from build123d import *

# Parameters (mm, degrees)
F2_R     = 1
F3_DEPTH = 10
F4_W     = 0.5
F4_H     = 4
F5_DEPTH = 30.001


with BuildPart() as f1:
    # F0 (on Right) → F1 (revolve)
    with BuildSketch(Plane.YZ):
        Polygon((5.690518, 7.5), (-0.309482, 7.5), (-0.309482, 5), (-10.309482, 5), (-10.309482, 0), (19.690518, 0), (19.690518, 7.5), (9.690518, 7.5), (9.690518, 4.5), (8.190518, 4.5), (8.190518, 7.5), (7.190518, 7.5), (7.190518, 4.5), (5.690518, 4.5), align=None)
    revolve(axis=Axis((0, 12.775562, 0), (0, 1, 0)))

    # F2 (on face) → F3 (cut)
    with BuildSketch(Plane.XZ.offset(10.309482)):
        with Locations((-2.5, 2)):
            Circle(F2_R)
        with Locations((2.5, 2)):
            Circle(F2_R)
        with Locations((-2.5, -2)):
            Circle(F2_R)
        with Locations((2.5, -2)):
            Circle(F2_R)
    extrude(amount=-F3_DEPTH, mode=Mode.SUBTRACT)

    # F4 (on face) → F5 (cut, through all)
    with BuildSketch(Plane.XZ.offset(10.309482)):
        with Locations((-0.25, 5.5)):
            Rectangle(F4_W, F4_H)
        with Locations((0.25, 5.5)):
            Rectangle(F4_W, F4_H)
    extrude(amount=-F5_DEPTH, mode=Mode.SUBTRACT)


solid = f1.part
Check sheet for the modelled part. Datum: model origin and axes. Units: mm. A direction names the side the tool comes from. Coordinates: 2 decimals unless noted, no trailing zeros. Write each loop counter-clockwise with the first axis right and the second up, starting at its lowest first coordinate (ties: lowest second). Pieces come first, ordered by that corner, then holes. Notation, with made-up numbers: M -21,-4.75 L 7,-4.75 A23 cw 7,11.25 Z; hole C 58.25,-39.75 d6. An arc over 180 degrees is marked long. Answer as CSV lines item,"result".
Q1. Cross-section at A-A (x = 0). Record the boundary of the cut face in (y, z), then the cut area to 3 significant figures.
Check result:
outline,"M -10.31,-5 L -0.31,-5 L -0.31,-7.5 L 5.69,-7.5 L 5.69,-4.5 L 7.19,-4.5 L 7.19,-7.5 L 8.19,-7.5 L 8.19,-4.5 L 9.69,-4.5 L 9.69,-7.5 L 19.69,-7.5 L 19.69,3.5 L -10.31,3.5 Z"
area,"296 mm^2"
Q2. Go/stop test with flat-tipped pins: pin 1 (3 mm diameter, centred on y = 9, z = 5.5, fed in from -X); pin 2 (1.6 mm diameter, centred on x = -2.5, z = -2, fed in from -Y); pin 3 (1.5 mm diameter, centred on x = 6, y = 4, fed in from +Z). Record where each tip stops, or that it passes through.
Check result:
pin 1,"x = -6.23"
pin 2,"y = -0.31"
pin 3,"z = 5.36"
Q3. Cross-section at B-B (y = -4). Record the boundary of the cut face in (x, z).
Check result:
outline,"M -0.5,3.5 L -0.5,4.97 A5 ccw long 0.5,4.97 L 0.5,3.5 Z; hole C -2.5,-2 d2; hole C -2.5,2 d2; hole C 2.5,-2 d2; hole C 2.5,2 d2"
Q4. Mould release check, pull along Y, two halves, no side actions. Record for faces 1 (the face through (-2, -0.309, 5)), 2 (the face through (-3.2, 7.191, -3.4)), 3 (the face through (-3.3, -5.4, -2.6)): released by +Y, released by -Y, zero draft, split by the parting line, or undercut.
Check result:
face 1,"released by -Y"
face 2,"undercut"
face 3,"zero draft"
Q5. Material ranges on probe 1 along Y at (x, z) = (-2.5, 4.5); probe 2 along Y at (x, z) = (1, -4.5); probe 3 along Z at (x, y) = (-2.5, -4.5), recorded low to high. Write a range as from..to.
Check result:
probe 1,"-0.31..5.69, 7.19..8.19, 9.69..19.69"
probe 2,"-10.31..5.69, 7.19..8.19, 9.69..19.69"
probe 3,"-4.33..-3, -1..1, 3..4.33"
Q6. Cross-section at D-D (z = 0). Record the boundary of the cut face in (x, y), then the cut area to 3 significant figures.
Check result:
outline,"M -7.5,-0.31 L -5,-0.31 L -5,-10.31 L 5,-10.31 L 5,-0.31 L 7.5,-0.31 L 7.5,5.69 L 4.5,5.69 L 4.5,7.19 L 7.5,7.19 L 7.5,8.19 L 4.5,8.19 L 4.5,9.69 L 7.5,9.69 L 7.5,19.69 L -7.5,19.69 L -7.5,9.69 L -4.5,9.69 L -4.5,8.19 L -7.5,8.19 L -7.5,7.19 L -4.5,7.19 L -4.5,5.69 L -7.5,5.69 Z"
area,"382 mm^2"
Q7. Set-up check for faces 4 (the face through (0.323, 2.649, -7.493)), 5 (the face through (0, 4, 3.5)), 6 (the face through (2, -0.309, -2)), 7 (the face through (-3.2, 9.691, -3.4)): record each of +Z, -Z, +X, -X, +Y, -Y from which the full face is reachable in a straight line by a thin tool's end or side.
Check result:
face 4,"+Y, -Y"
face 5,"+Z, +Y, -Y"
face 6,"-Y"
face 7,"none"
Q8. Cross-section at C-C (z = -6.5). Record the boundary of the cut face in (x, y), then the cut area to 3 significant figures.
Check result:
outline,"M -3.74,-0.31 L 3.74,-0.31 L 3.74,5.69 L -3.74,5.69 Z; M -3.74,7.19 L 3.74,7.19 L 3.74,8.19 L -3.74,8.19 Z; M -3.74,9.69 L 3.74,9.69 L 3.74,19.69 L -3.74,19.69 Z"
area,"127 mm^2"
